Read the model definition and answer for the solid it produces. Units are mm, in the model's axes. Coordinates: 2 decimals unless noted, no trailing zeros. Write each loop counter-clockwise with the first axis right and the second up, starting at its lowest first coordinate (ties: lowest second). Pieces come first, ordered by that corner, then holes. Notation, with made-up numbers: (-38.75, 57.5) -> (-10.75, 57.5) arc R28 cw to (-10.75, 96.5) -> close; hole circle Ø2 at (-26.75, 9). An arc over 180 degrees is marked (long way). Write item = value, one per line. Start each with the question number.
1) Section A-A (y = 0) is taken. Determine the outline of the cut face in (x, z), plus the area to 3 significant figures.
2) Find the intervals of material crossed by line 1 along X through (y, z) = (16, 8); line 2 along X through (y, z) = (21.5, 37.5); line 3 along Y through (x, z) = (-45.5, 20), in increasing order. Write a range as from..to.
3) Section B-B (z = 25) is taken. Determine the outline of the cut face in (x, y).
4) Flat-ended cylindrical pins translate along their axes: pin 1 Ø6 at (y, z) = (3.5, 29) entering from +X; pin 2 Ø12 at (y, z) = (11, 23) entering from +X; pin 3 Ø8 at (x, z) = (-29.5, 8.5) entering from -Y. Find the tip coordinate at first contact, or state that the pin passes through.
5) Section C-C (z = 9) is taken. Determine the outline of the cut face in (x, y), plus the area to 3 significant figures.
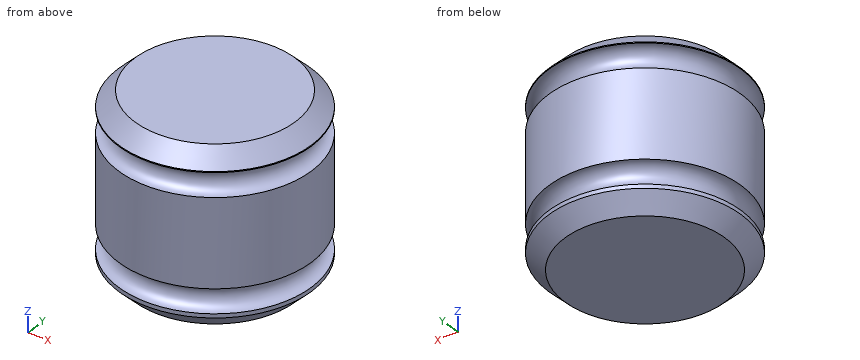
from build123d import *

# Parameters (mm, degrees)
F2_SIZE = 5.08


with BuildPart() as f1:
    # F0 (on Front) → F1 (revolve)
    with BuildSketch(Plane.XZ):
        with BuildLine():
            Line((-30.36179, 0), (0, 0))
            Line((0, 0), (0, 6.348697))
            ThreePointArc((0, 6.348697), (-3.7719, 10.120597), (0, 13.892497))
            Line((0, 13.892497), (0, 41.490039))
            ThreePointArc((0, 41.490039), (-3.766214, 45.256253), (0, 49.022468))
            Line((0, 49.022468), (0, 54.422077))
            Line((0, 54.422077), (-30.36179, 54.422077))
            Line((-30.36179, 54.422077), (-30.36179, 0))
        make_face()
    revolve(axis=Axis((-30.36179, 0, 27.211038), (0, 0, 1)))

    # F2
    f2_edges = [f1.edges().sort_by_distance(p)[0] for p in [
        (-60.72358, 0, 54.422077),
        (-60.72358, 0, 0),
    ]]
    chamfer(f2_edges, length=F2_SIZE)


solid = f1.part
Answer key:
q1.outline = (-60.72, 5.08) -> (-55.64, 0) -> (-5.08, 0) -> (0, 5.08) -> (0, 6.35) arc R3.77 cw to (0, 13.89) -> (0, 41.49) arc R3.77 cw to (0, 49.02) -> (0, 49.34) -> (-5.08, 54.42) -> (-55.64, 54.42) -> (-60.72, 49.34) -> (-60.72, 49.02) arc R3.77 cw to (-60.72, 41.49) -> (-60.72, 13.89) arc R3.77 cw to (-60.72, 6.35) -> close
q1.area = 3,160 mm^2
q2.line_1 = -52.41..-8.31
q2.line_2 = -51.8..-8.92
q2.line_3 = -26.32..26.32
q3.outline = circle Ø60.72 at (-30.36, 0)
q4.pin_1 = 0
q4.pin_2 = -0.41
q4.pin_3 = -30.36
q5.outline = circle Ø53.52 at (-30.36, 0)
q5.area = 2,250 mm^2
